```python
from build123d import *

# Parameters (mm, degrees)
SCHIZZO1_W                   = 106.2
SCHIZZO1_H                   = 33.2
ESTRUSIONE_ESTRUSIONE1_DEPTH = 55.2
RACCORDO1_R                  = 2
SCHIZZO2_W                   = 12
SCHIZZO2_H                   = 13
ESTRUSIONE_ESTRUSIONE2_DEPTH = 6
SMUSSO1_SIZE2                = 10
SMUSSO1_SIZE                 = 6
SCHIZZO4_W                   = 9.15
SCHIZZO4_H                   = 7.5
ESTRUSIONE_ESTRUSIONE3_DEPTH = 2.8
SMUSSO2_SIZE2                = 6
SMUSSO2_SIZE                 = 2.8
SCHIZZO5_W                   = 25.4
SCHIZZO5_H                   = 16
ESTRUSIONE_ESTRUSIONE4_DEPTH = 2.5


with BuildPart() as part:
    # Schizzo1 → Estrusione-Estrusione1 (new body)
    with BuildSketch(Plane.XY):
        with Locations((1.864332707, 11.26679198)):
            Rectangle(SCHIZZO1_W, SCHIZZO1_H)
    extrude(amount=ESTRUSIONE_ESTRUSIONE1_DEPTH)

    # Raccordo1
    raccordo1_edges = [part.edges().sort_by_distance(p)[0] for p in [
        (54.964332707, 11.26679198, 55.2),
        (1.864332707, 27.86679198, 55.2),
        (-51.235667293, 11.26679198, 55.2),
        (1.864332707, 27.86679198, 0),
        (54.964332707, 11.26679198, 0),
        (1.864332707, -5.33320802, 0),
        (-51.235667293, 11.26679198, 0),
        (1.864332707, -5.33320802, 55.2),
        (-51.235667293, 27.86679198, 27.6),
        (54.964332707, 27.86679198, 27.6),
        (54.964332707, -5.33320802, 27.6),
        (-51.235667293, -5.33320802, 27.6),
    ]]
    fillet(raccordo1_edges, radius=RACCORDO1_R)

    # Schizzo2 → Estrusione-Estrusione2 (add)
    with BuildSketch(Plane.ZY.offset(51.235667293)):
        with Locations((42, 13.16679198)):
            Rectangle(SCHIZZO2_W, SCHIZZO2_H)
    extrude(amount=ESTRUSIONE_ESTRUSIONE2_DEPTH)

    # Smusso1
    smusso1_edges = [part.edges().sort_by_distance(p)[0] for p in [
        (-57.235667293, 6.66679198, 42),
    ]]
    smusso1_side = [part.faces().sort_by_distance(p)[0] for p in [
        (-57.115667293, 6.66679198, 42),
    ]]
    chamfer(smusso1_edges, length=SMUSSO1_SIZE - 0.0001, length2=SMUSSO1_SIZE2 - 0.0001, reference=smusso1_side[0])  # a hair under: the kernel refuses the full size

    # Schizzo4 → Estrusione-Estrusione3 (add)
    with BuildSketch(Plane(origin=(54.964332707, 0, 0), x_dir=(0, 0, -1), z_dir=(1, 0, 0))):
        with Locations((-21.425, 3.91679198)):
            Rectangle(SCHIZZO4_W, SCHIZZO4_H)
    extrude(amount=ESTRUSIONE_ESTRUSIONE3_DEPTH)

    # Smusso2
    smusso2_edges = [part.edges().sort_by_distance(p)[0] for p in [
        (57.764332707, 0.16679198, 21.425),
    ]]
    smusso2_side = [part.faces().sort_by_distance(p)[0] for p in [
        (57.708332707, 0.16679198, 21.425),
    ]]
    chamfer(smusso2_edges, length=SMUSSO2_SIZE - 0.0001, length2=SMUSSO2_SIZE2 - 0.0001, reference=smusso2_side[0])  # a hair under: the kernel refuses the full size

    # Schizzo5 → Estrusione-Estrusione4 (add)
    with BuildSketch(Plane(origin=(0, 0, 0), x_dir=(-1, 0, 0), z_dir=(0, 0, -1))):
        with Locations((31.935667293, 15.86679198)):
            Rectangle(SCHIZZO5_W, SCHIZZO5_H)
    extrude(amount=ESTRUSIONE_ESTRUSIONE4_DEPTH)


solid = part.part
```
Can you work these out from the model? Positions are in its coordinate system, mm. A direction names the side the tool comes from. Round coordinates to 2 decimals unless told otherwise and drop trailing zeros. Loops run counter-clockwise (first coordinate to the right, second up) from the corner with the lowest first, then second, coordinate; pieces in that order, holes last.
Item 1: Suppose I cut it at C-C, the plane y = 22.5. Write out the boundary of the cut face in (x, z).
Item 2: Will these pins go through, and if not, where does the flat tip stop? pin 1 Ø12 at (y, z) = (11.5, 32) entering from +X; pin 2 Ø0.8 at (x, z) = (-27.5, -2) entering from -Y; pin 3 Ø1.2 at (y, z) = (17.5, -1) entering from -X.
Item 3: Suppose I cut it at B-B, the plane x = -35. Write out the boundary of the cut face in (y, z).
Item 4: Suppose I cut it at A-A, the plane z = 7. Write out the boundary of the cut face in (x, y), then the cut area to 3 significant figures.
Item 5: Please list where these lines run through material, in increasing order: L1, parallel to Z at x = -14, y = 17.5; L2, parallel to X at y = 21, z = 10; L3, parallel to Y at x = -46, z = 53.5.
Item 6: Which directions (+Z, -Z, +X, -X, +Y, -Y) give clear straight access to the entire face, cutting with the end or side of a thin tool? Please do faces 1 (the flat face through (-44.636, 16, -1)), 2 (the flat face through (-54, 15, 48)), 3 (the flat face through (56, 7.667, 21)), 4 (the flat face through (-19.236, 16, -1)).
Reported:
1. outline: (-51.24, 2) arc R2 ccw to (-49.24, 0) - (-44.64, 0) - (-44.64, -2.5) - (-19.24, -2.5) - (-19.24, 0) - (52.96, 0) arc R2 ccw to (54.96, 2) - (54.96, 53.2) arc R2 ccw to (52.96, 55.2) - (-49.24, 55.2) arc R2 ccw to (-51.24, 53.2) - close
2. pin 1: stops at x = 54.96
2. pin 2: stops at y = 7.87
2. pin 3: stops at x = -44.64
3. outline: (-5.33, 2) arc R2 ccw to (-3.33, 0) - (7.87, 0) - (7.87, -2.5) - (23.87, -2.5) - (23.87, 0) - (25.87, 0) arc R2 ccw to (27.87, 2) - (27.87, 53.2) arc R2 ccw to (25.87, 55.2) - (-3.33, 55.2) arc R2 ccw to (-5.33, 53.2) - close
4. outline: (-51.24, -3.33) arc R2 ccw to (-49.24, -5.33) - (52.96, -5.33) arc R2 ccw to (54.96, -3.33) - (54.96, 25.87) arc R2 ccw to (52.96, 27.87) - (-49.24, 27.87) arc R2 ccw to (-51.24, 25.87) - close
4. area: 3,520 mm2
5. L1: z = 0 to 55.2
5. L2: x = -51.24 to 54.96
5. L3: y = -5.31 to 27.84
6. face 1: -Z, -X, +Y, -Y
6. face 2: +Z, -X, +Y, -Y
6. face 3: +Z, -Z, +X, +Y
6. face 4: -Z, +X, +Y, -Y
